```python
from build123d import *

# Parameters (mm, degrees)
F1_DEPTH = 153
F3_DEPTH = 30
F4_R     = 1
F6_R     = 0.5
F7_R     = 0.5


# Not quite as in the source:
# - two fillets or chamfers of one size are made in one step
# - a pattern or mirror of a feature is missing from the dataset's text; its kind, count and spacing are read off the source's solid


with BuildPart() as f1:
    # F0 (on Top) → F1 (new body, symmetric)
    with BuildSketch(Plane.XY):
        Polygon((-14, 0.5), (-17, 0.5), (-20, -2.5), (20, -2.5), (17, 0.5), (14, 0.5), (11, 0.5), (-11, 0.5), align=None)
        Polygon((-14, 25.5), (-14, 0.5), (-11, 0.5), (-11, 4), (-11, 7), (-11, 25.5), align=None)
        Polygon((11, 4), (11, 0.5), (14, 0.5), (14, 25.5), (11, 25.5), (11, 7), align=None)
        Polygon((-11, 7), (-11, 4), (-5, 4), (-5, 7), (-5, 15), (-8, 15), (-8, 7), align=None)
        Polygon((5, 4), (11, 4), (11, 7), (8, 7), (8, 15), (5, 15), (5, 7), align=None)
    extrude(amount=F1_DEPTH, both=True)

    # F2 (on Right) → F3 (cut, symmetric)
    with BuildSketch(Plane.YZ):
        Polygon((25.5, 153), (0.5, 153), (-2.5, 153), (25.5, 125), align=None)
    f3 = extrude(amount=F3_DEPTH, both=True, mode=Mode.SUBTRACT)

    # F3_copies: F3 across plane
    add(f3.mirror(Plane(origin=(0, 0, 0), x_dir=(-1, 0, 0), z_dir=(0, 0, -1))), mode=Mode.SUBTRACT)

    # F4
    f4_edges = [f1.edges().sort_by_distance(p)[0] for p in [
        (17, 0.5, 0),
        (12.5, 25.5, 125),
        (-11, 0.5, 0),
        (-12.5, 25.5, 125),
        (-17, 0.5, 0),
        (11, 0.5, 0),
        (6.5, 15, 135.5),
        (-6.5, 15, 135.5),
        (12.5, 25.5, -125),
        (6.5, 15, -135.5),
        (-6.5, 15, -135.5),
        (-12.5, 25.5, -125),
        (5, 4, 0),
        (-5, 4, 0),
    ]]
    fillet(f4_edges, radius=F4_R)

    # F6
    f6_edges = [f1.edges().sort_by_distance(p)[0] for p in [
        (-8, 7, 0),
        (-11, 7, 0),
        (-11, 4, 0),
        (11, 4, 0),
        (11, 7, 0),
        (8, 7, 0),
    ]]
    fillet(f6_edges, radius=F6_R)

    # F7
    f7_edges = [f1.edges().sort_by_distance(p)[0] for p in [
        (20, -2.5, 0),
        (-20, -2.5, 0),
    ]]
    fillet(f7_edges, radius=F7_R)


solid = f1.part
```
Read the model definition and answer for the solid it produces. Units are mm, in the model's axes. A direction names the side the tool comes from. Round coordinates to 2 decimals unless told otherwise and drop trailing zeros. Write each loop counter-clockwise with the first axis right and the second up, starting at its lowest first coordinate (ties: lowest second). Pieces come first, ordered by that corner, then holes. Notation, with made-up numbers: M 73.5,-35 L 108.5,-35 A22 ccw 108.5,3 Z; hole C -1.75,-9.75 d11. An arc over 180 degrees is marked long. One line per item, written item: value.
Q1. Find section A-A on y = 11.25. Write down the section's boundary in (x, z).
Data:
outline: M -14,-139.25 L -11,-139.25 L -11,139.25 L -14,139.25 Z; M -8,-139.25 L -5,-139.25 L -5,139.25 L -8,139.25 Z; M 5,-139.25 L 8,-139.25 L 8,139.25 L 5,139.25 Z; M 11,-139.25 L 14,-139.25 L 14,139.25 L 11,139.25 Z
Q2. Straight lines are drawn through the part: line 1 (X direction, y = 13.5, z = -114); line 2 (X direction, y = 15.75, z = -129); line 3 (Y direction, x = 9, z = -107). For each, find the intervals that lie inside material, in ascending order. Write a range as [from, to].
Data:
line 1: [-14, -11], [-8, -5], [5, 8], [11, 14]
line 2: [-14, -11], [11, 14]
line 3: [-2.5, 0.5], [4, 7]
Q3. Which of the six approach directions +Z, -Z, +X, -X, +Y, -Y give full straight-line access (tool end or side, diameter ignored) to faces 1 (the flat face through (0, 0.5, 2)), 2 (the flat face through (5, 10, 2)), 3 (the flat face through (0, -2.5, 2))?
Data:
face 1: +Z, -Z
face 2: +Z, -Z, +Y
face 3: +Z, -Z, +X, -X, -Y
Q4. For a pull along X with two mould halves and no side action, classify faces 4 (the flat face through (-14, 13, 2)), 5 (the flat face through (5.8, 6.2, -144.3)), 6 (the flat face through (-8, 11, 2)), 7 (the flat face through (14, 13, 2)) as +X half, -X half, draft (parallel to the pull), parting line (faces both ways), or undercut.
Data:
face 4: -X half
face 5: draft
face 6: undercut
face 7: +X half
Q5. Flat-ended cylindrical pins translate along their axes: pin 1 Ø3 at (x, z) = (2, 24) entering from +Y; pin 2 Ø5 at (y, z) = (12, 59.5) entering from +X; pin 3 Ø14.5 at (y, z) = (16.5, 21) entering from -X. Find the tip coordinate at first contact, or state that the pin passes through.
Data:
pin 1: y = 0.5
pin 2: x = 14
pin 3: x = -14
